from build123d import *

# Parameters (mm, degrees)
SKETCH015_W     = 127
SKETCH015_H     = 28
PAD006_DEPTH    = 6.8
SKETCH016_W     = 1.5
SKETCH016_H     = 6.8
PAD007_DEPTH    = 1.5
SKETCH017_W     = 1.5
SKETCH017_H     = 6.8
PAD008_DEPTH    = 1.5
SKETCH018_R     = 3.03
POCKET007_DEPTH = 6.801
SKETCH019_R     = 1.05
SKETCH019_R_2   = 1.5
POCKET008_DEPTH = 29.501
SKETCH020_W     = 101
SKETCH020_H     = 5.7
POCKET009_DEPTH = 1.69
SKETCH022_W     = 5
SKETCH022_H     = 3.4
PAD010_DEPTH    = 7


with BuildPart() as pocket009:
    # Sketch015 → Pad006 (new body)
    with BuildSketch(Plane.XY):
        with Locations((-63.932219, -3.966905)):
            Rectangle(SKETCH015_W, SKETCH015_H)
    extrude(amount=PAD006_DEPTH)

    # Sketch016 → Pad007 (new body)
    with BuildSketch(Plane.XZ.offset(17.966905)):
        with Locations((-126.682219, 3.4)):
            Rectangle(SKETCH016_W, SKETCH016_H)
    extrude(amount=PAD007_DEPTH)

    # Sketch017 → Pad008 (new body)
    with BuildSketch(Plane(origin=(0, 10.033095, 0), x_dir=(-1, 0, 0), z_dir=(0, 1, 0))):
        with Locations((126.682219, 3.4)):
            Rectangle(SKETCH017_W, SKETCH017_H)
    extrude(amount=PAD008_DEPTH)

    # Sketch018 → Pocket007 (cut, through all)
    with BuildSketch(Plane.XY.offset(6.8)):
        with Locations((-56.432219, -3.966905)):
            Circle(SKETCH018_R)
    extrude(amount=-POCKET007_DEPTH, mode=Mode.SUBTRACT)

    # Sketch019 → Pocket008 (cut, through all)
    with BuildSketch(Plane.XZ.offset(17.966905)):
        with Locations((-56.432219, 3.4)):
            Circle(SKETCH019_R)
        with Locations((-117.432219, 3.4)):
            Circle(SKETCH019_R_2)
        with Locations((-34.475986, 3.4)):
            Circle(SKETCH019_R_2)
    extrude(amount=-POCKET008_DEPTH, mode=Mode.SUBTRACT)

    # Sketch020 → Pocket009 (cut)
    with BuildSketch(Plane(origin=(0, 0, 0), x_dir=(1, 0, 0), z_dir=(0, 0, -1))):
        with Locations((-50.932219, 11.516905)):
            Rectangle(SKETCH020_W, SKETCH020_H)
    extrude(amount=-POCKET009_DEPTH, mode=Mode.SUBTRACT)


with BuildPart() as pad010:
    # Part__Mirroring: instance of Pocket009
    add(pocket009.part.mirror(Plane(origin=(0, 0, 0), x_dir=(0, -1, 0), z_dir=(1, 0, 0))))

    # Sketch022 → Pad010 (new body)
    with BuildSketch(Plane(origin=(0.432219, 0, 0), x_dir=(0, -1, 0), z_dir=(-1, 0, 0))):
        with Locations((-4.533095, 5.1)):
            Rectangle(SKETCH022_W, SKETCH022_H)
        with Locations((12.466905, 5.1)):
            Rectangle(SKETCH022_W, SKETCH022_H)
    extrude(amount=PAD010_DEPTH)


solid = pad010.part
For this review, take the finished solid that the model builds, in its own axes (mm). A direction names the side the tool comes from. Give positions to 0.01 mm unless a question says otherwise; leave off trailing zeros. Loops run counter-clockwise (first coordinate to the right, second up) from the corner with the lowest first, then second, coordinate; pieces in that order, holes last.
Item 1: Tool access review of faces 5 (the flat face through (-3, 2.033, 5)), 6 (the flat face through (64, -17.967, 3)), 7 (the flat face through (64, 10.033, 3)): name each direction out of +Z, -Z, +X, -X, +Y, -Y from which nothing blocks a thin tool from reaching the whole face with its end or side.
Item 2: Take a section at A-A, the plane y = 0.5. State the section outline as (x, z) points.
Item 3: Draft analysis for pull direction X (two halves, no side actions). For faces 1 (the flat face through (127.432, -4, 3)), 2 (the flat face through (-3, -12, 3.4)), 3 (the flat face through (-6.568, 5, 5)), 4 (the cylindrical face through (53.633, -5.127, 3.448)), state which applies: +X half, -X half, draft (parallel to the pull), parting line (faces both ways), or undercut.
Item 4: Insertion check: pin 1 (1.5 mm diameter, centred on x = -3, y = 4.5, fed in from -Z); pin 2 (4 mm diameter, centred on x = 34.48, z = 3.4, fed in from -Y); pin 3 (3 mm diameter, centred on y = -14, z = 1.5, fed in from -X). Each pin has a flat end and moves straight along its axis. Give the tip position at first contact, or say it passes through.
Item 5: Take a section at B-B, the plane x = 93. State the section outline as (y, z) points, and give its area (3 significant figures).
Item 6: For line 1 along Y through (x, z) = (3, 0.5); line 2 along X through (y, z) = (8.5, 2.5); line 3 along X through (y, z) = (-14, 3.75), list the stretches that pass through material, from the lowest coordinate up.
Calculated:
1. face 5: +Z, -Z, -X
1. face 6: +Z, -Z, -X, -Y
1. face 7: +Z, -Z, -X, +Y
2. outline: (0.43, 0) - (127.43, 0) - (127.43, 6.8) - (0.43, 6.8) - close; hole circle Ø3 at (34.48, 3.4); hole circle Ø2.1 at (56.43, 3.4); hole circle Ø3 at (117.43, 3.4)
3. face 1: +X half
3. face 2: draft
3. face 3: -X half
3. face 4: undercut
4. pin 1: stops at z = 3.4
4. pin 2: stops at y = -17.97
4. pin 3: stops at x = 0.43
5. outline: (-17.97, 0) - (-14.37, 0) - (-14.37, 1.69) - (-8.67, 1.69) - (-8.67, 0) - (10.03, 0) - (10.03, 6.8) - (-17.97, 6.8) - close
5. area: 181 mm2
6. line 1: y = -17.97 to -14.37, -8.67 to 10.03
6. line 2: x = 0.43 to 33.28, 35.68 to 55.89, 56.97 to 116.23, 118.63 to 127.43
6. line 3: x = -6.57 to 33.02, 35.93 to 55.44, 57.42 to 115.97, 118.89 to 127.43
